```python
from build123d import *

# Parameters (mm, degrees)
SKETCH1_W               = 304.8
SKETCH1_H               = 127
BOSS_EXTRUDE1_DEPTH     = 3.175
SKETCH2_R               = 2.54
CUT_EXTRUDE1_DEPTH      = 166.130526024
CUT_EXTRUDE2_DEPTH      = 166.130526024
CUT_EXTRUDE2_DEPTH_BACK = 166.130526024
SKETCH3_R               = 2


with BuildPart() as part:
    # Sketch1 → Boss-Extrude1 (new body)
    with BuildSketch(Plane.XY):
        Rectangle(SKETCH1_W, SKETCH1_H)
    extrude(amount=BOSS_EXTRUDE1_DEPTH)

    # Sketch2 → Cut-Extrude1 (cut, through all)
    with BuildSketch(Plane.XY.offset(3.175)):
        with Locations((50.8, 19.05)):
            Circle(SKETCH2_R)
        with Locations((50.8, -19.05)):
            Circle(SKETCH2_R)
        with Locations((-50.8, -19.05)):
            Circle(SKETCH2_R)
        with Locations((-50.8, 19.05)):
            Circle(SKETCH2_R)
    extrude(amount=-CUT_EXTRUDE1_DEPTH, mode=Mode.SUBTRACT)

    # Sketch3 → Cut-Extrude2 (cut, two sides: drawn at the far end of the back side and taken through both)
    with BuildSketch(Plane(origin=(0, 0, 0), x_dir=(-1, 0, 0), z_dir=(0, 0, -1)).offset(-CUT_EXTRUDE2_DEPTH_BACK)):
        with Locations((-20.5, 12.5)):
            Circle(SKETCH3_R)
        with Locations((20.5, -12.5)):
            Circle(SKETCH3_R)
        with Locations((20.5, 12.5)):
            Circle(SKETCH3_R)
        with Locations((-20.5, -12.5)):
            Circle(SKETCH3_R)
        Polygon((11.27, 21.395), (11.27, -21.395), (-11.27, -21.395), (-11.27, 21.395), (-3.81, 21.395), (-3.81, 29.015), (3.81, 29.015), (3.81, 21.395), align=None)
    extrude(amount=CUT_EXTRUDE2_DEPTH + CUT_EXTRUDE2_DEPTH_BACK, mode=Mode.SUBTRACT)


solid = part.part
```
Check sheet for the modelled part. Datum: model origin and axes. Units: mm. Coordinates: 2 decimals unless noted, no trailing zeros.
1) Material ranges on probe 1 along Y at (x, z) = (-50.8, 0.7); probe 2 along Y at (x, z) = (20.5, 1.75); probe 3 along X at (y, z) = (-12.5, 1.65), recorded low to high.
2) Gauge pin test, flat end, axial feed: pin 1 (3 mm diameter, centred on x = 20.5, y = 12.5, fed in from -Z). Record the tip position at first contact, or that the pin passes through.
3) Release check for a two-part mould opening along X. For faces 1 (the face through (53.223, -18.287, 1.61)), 2 (the face through (-2, -27, 0)), 3 (the face through (-48.377, -18.287, 1.61)) record: released by +X, released by -X, zero draft, split by the parting line, or undercut.
4) Sectioned sample at A-A (z = 2.15). Count the separate pieces of the cut face and the enclosed holes in it, and give its area (3 significant figures).
Check sheet entries:
1. probe 1: y = -63.5 to -21.59, -16.51 to 16.51, 21.59 to 63.5
1. probe 2: y = -63.5 to -14.5, -10.5 to 10.5, 14.5 to 63.5
1. probe 3: x = -152.4 to -22.5, -18.5 to -11.27, 11.27 to 18.5, 22.5 to 152.4
2. pin 1: passes through
3. face 1: undercut
3. face 2: zero draft
3. face 3: undercut
4. separate pieces: 1
4. enclosed holes: 9
4. area: 37,600 mm2
